from build123d import *

# Parameters (mm, degrees)
SKETCH1_W                      = 57.15
SKETCH1_H                      = 31.75
BOSS_EXTRUDE1_DEPTH            = 3.175
M4_CLEARANCE_HOLE1_D           = 4.5
M4_CLEARANCE_HOLE1_CSINK_D     = 4.55
M4_CLEARANCE_HOLE1_CSINK_ANGLE = 90
SKETCH5_W                      = 12.7
SKETCH5_H                      = 37.846
BOSS_EXTRUDE2_DEPTH            = 9.525
BOSS_EXTRUDE3_DEPTH            = 9.525
M4_CLEARANCE_HOLE2_D           = 4.5
M4_CLEARANCE_HOLE2_DEPTH       = 33.02
M4_CLEARANCE_HOLE2_CSINK_D     = 4.55
M4_CLEARANCE_HOLE2_CSINK_ANGLE = 90
M4_CLEARANCE_HOLE2_TIP         = 1.351936393


with BuildPart() as part:
    # Sketch1 → Boss-Extrude1 (new body)
    with BuildSketch(Plane(origin=(0, 0, 0), x_dir=(1, 0, 0), z_dir=(0, 1, 0))):
        Rectangle(SKETCH1_W, SKETCH1_H)
    extrude(amount=BOSS_EXTRUDE1_DEPTH)

    # M4 Clearance Hole1 (through all)
    with Locations(Plane(origin=(0, 3.175, 0), x_dir=(1, 0, 0), z_dir=(0, 1, 0))):
        with Locations((-19.05, 9.525), (19.05, 9.525), (19.05, -9.525), (-19.05, -9.525)):
            CounterSinkHole(M4_CLEARANCE_HOLE1_D / 2, M4_CLEARANCE_HOLE1_CSINK_D / 2, counter_sink_angle=M4_CLEARANCE_HOLE1_CSINK_ANGLE)

    # Sketch5 → Boss-Extrude2 (add, symmetric)
    with BuildSketch(Plane.XY):
        with Locations((0, 22.098)):
            Rectangle(SKETCH5_W, SKETCH5_H)
    extrude(amount=BOSS_EXTRUDE2_DEPTH, both=True)

    # Sketch6 → Boss-Extrude3 (add, symmetric)
    with BuildSketch(Plane.XY):
        Polygon((6.35, 41.021), (12.7, 41.021), (12.7, 67.691), (22.86, 67.691), (22.86, 34.671), (15.175054079, 34.671), (6.35, 25.845945921), align=None)
        Polygon((-6.35, 41.021), (-12.7, 41.021), (-12.7, 67.691), (-22.86, 67.691), (-22.86, 34.671), (-15.175054079, 34.671), (-6.35, 25.845945921), align=None)
        Polygon((-6.35, 10.795), (-13.97, 3.175), (-6.35, 3.175), align=None)
        Polygon((6.35, 3.175), (6.35, 10.795), (13.97, 3.175), align=None)
    extrude(amount=BOSS_EXTRUDE3_DEPTH, both=True)

    # M4 Clearance Hole2
    with Locations(Plane(origin=(0, 67.691, 0), x_dir=(1, 0, 0), z_dir=(0, 1, 0))):
        with Locations((-17.903194087, 0), (17.656805913, 0)):
            CounterSinkHole(M4_CLEARANCE_HOLE2_D / 2, M4_CLEARANCE_HOLE2_CSINK_D / 2, depth=M4_CLEARANCE_HOLE2_DEPTH, counter_sink_angle=M4_CLEARANCE_HOLE2_CSINK_ANGLE)
            with Locations((0, 0, -(M4_CLEARANCE_HOLE2_DEPTH + M4_CLEARANCE_HOLE2_TIP / 2))):  # 118° drill point
                Cone(0, M4_CLEARANCE_HOLE2_D / 2, M4_CLEARANCE_HOLE2_TIP, mode=Mode.SUBTRACT)


solid = part.part
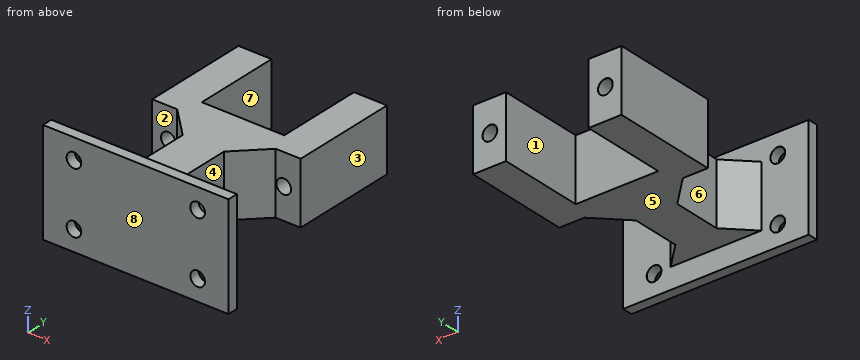
Geometry check sheet. Reference: the model listing, model coordinates, mm. Face numbers are marked on the shaded views. A direction names the side the tool comes from. Give positions to 0.01 mm unless a question says otherwise; leave off trailing zeros. Loops run counter-clockwise (first coordinate to the right, second up) from the corner with the lowest first, then second, coordinate; pieces in that order, holes last. Notation, with made-up numbers: (67.5, -20) -> (96.5, -20) arc R20 cw to (96.5, 13) -> close; hole circle Ø7 at (22.5, 29). An arc over 180 degrees is marked (long way). Answer in a Markdown table with one row per item. Add a question column.
1) Cross-section at C-C on x = 5. Record the boundary of the cut face in (y, z) (3 decimals), and give its area (3 significant figures).
2) Cross-section at B-B on z = 0. State how many separate pieces and enclosed holes the cut face has, and give its area (3 significant figures).
3) Cross-section at D-D on y = 38. Record the boundary of the cut face in (x, z) (3 decimals), and give its area (3 significant figures).
4) Set-up check for the marked faces 1, 2, 3, 4 and 5: record each of +Z, -Z, +X, -X, +Y, -Y from which the full face is reachable in a straight line by a thin tool's end or side.
5) Cross-section at A-A on y = 49.5. Record the boundary of the cut face in (x, z) (3 decimals).
6) Material ranges on probe 1 along Z at (x, y) = (-19, 1) (3 decimals); probe 2 along Y at (x, z) = (22, 2) (3 decimals); probe 3 along Y at (x, z) = (-25, 5.5) (3 decimals), recorded low to high. Write a range as from..to.
7) Gauge pin test, flat ends, axial feed: P1, Ø2.5, axis at x = 19.05, z = 9.525, coming from the -Y side; P2, Ø1.5, axis at x = 1.5, y = 23, coming from the -Z side (3 decimals); P3, Ø15, axis at y = 55.5, z = 2, coming from the +X side. Record the tip position at first contact, or that the pin passes through.
8) Draft check along Y on the marked faces 6, 7 and 8. Enter one of: pulls with the +Y half, pulls with the -Y half, needs draft (parallel to the pull), parting line crosses it, or undercut.
Outcome:
| question | item | result |
|---|---|---|
| 1 | outline | (0, -15.875) -> (3.175, -15.875) -> (3.175, -9.525) -> (41.021, -9.525) -> (41.021, 9.525) -> (3.175, 9.525) -> (3.175, 15.875) -> (0, 15.875) -> close |
| 1 | area | 822 mm^2 |
| 2 | separate pieces | 3 |
| 2 | enclosed holes | 0 |
| 2 | area | 1,250 mm^2 |
| 3 | outline | (-22.86, -9.525) -> (22.86, -9.525) -> (22.86, 9.525) -> (-22.86, 9.525) -> close; hole circle Ø4.5 at (-17.903, 0); hole circle Ø4.5 at (17.657, 0) |
| 3 | area | 839 mm^2 |
| 4 | face 1 | +Z, -Z, +Y |
| 4 | face 2 | +Z, -Z, -X |
| 4 | face 3 | +Z, -Z, +X, +Y |
| 4 | face 4 | +Z, -Z, +X |
| 4 | face 5 | -Z, +X, -X, +Y |
| 5 | outline | (-22.86, -9.525) -> (-12.7, -9.525) -> (-12.7, 9.525) -> (-22.86, 9.525) -> close; (12.7, -9.525) -> (22.86, -9.525) -> (22.86, 9.525) -> (12.7, 9.525) -> close; hole circle Ø4.5 at (-17.903, 0); hole circle Ø4.5 at (17.657, 0) |
| 6 | probe 1 | z = -15.875..-11.774, -7.276..7.276, 11.774..15.875 |
| 6 | probe 2 | y = 0..3.175, 34.671..67.691 |
| 6 | probe 3 | y = 0..3.175 |
| 7 | P1 | stops at y = 34.67 |
| 7 | P2 | stops at z = -9.525 |
| 7 | P3 | stops at x = 22.86 |
| 8 | face 6 | undercut |
| 8 | face 7 | needs draft |
| 8 | face 8 | pulls with the -Y half |
